Input: dimensioned drawing with shaded views. Units: mm. Origin: part minimum x, y, z. Coordinates: 2 decimals unless noted, no trailing zeros.
Item 1: Pull-direction query (X, two-part tool) for the marked faces 1, 2 and 3; classes: +X half, -X half, draft (parallel to the pull), parting line (faces both ways), or undercut.
Item 2: Pin query (flat end, axial travel): pin 1 Ø10 at (y, z) = (35, 21) entering from -X. Return the tip coordinate at first contact, or that it passes through.
Item 3: Line query: probe 1 along Y at (x, z) = (97.5, 23). Output: solid intervals per line, ascending.
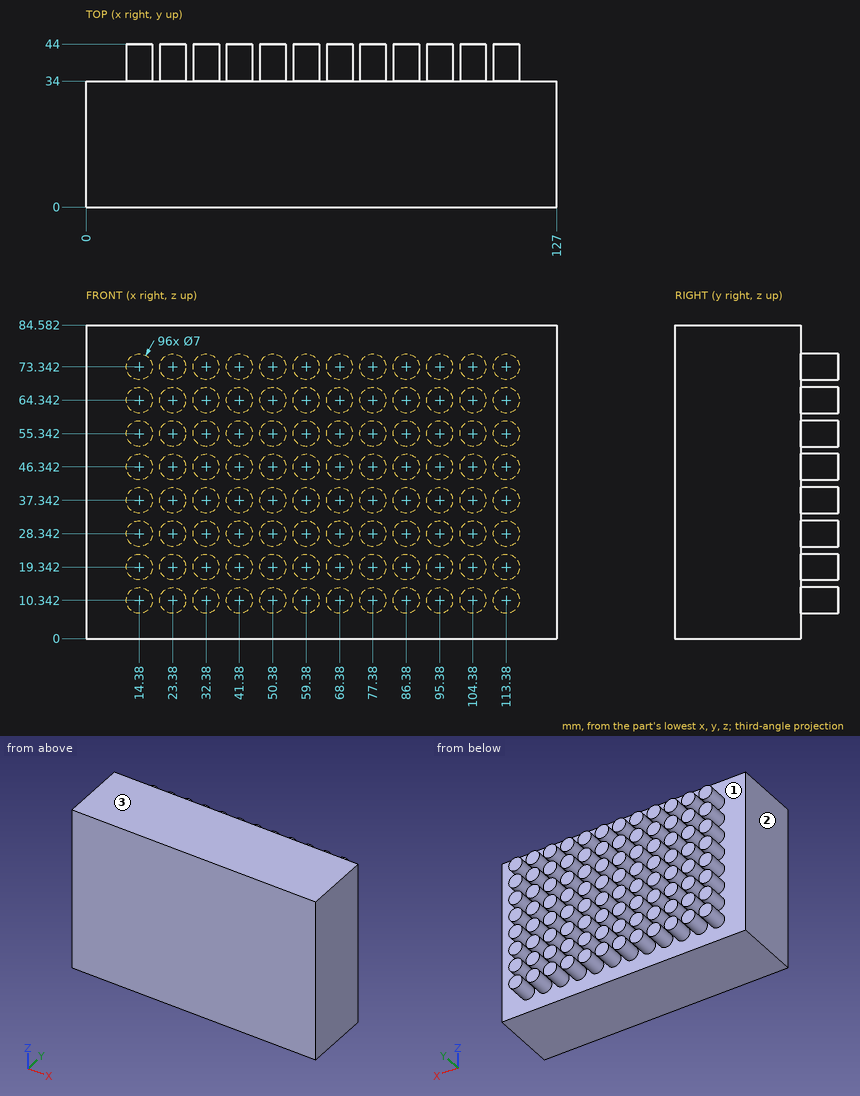
Verdict:
1. face 1: undercut
1. face 2: -X half
1. face 3: draft
2. pin 1: stops at x = 0
3. probe 1: y = 0 to 34
